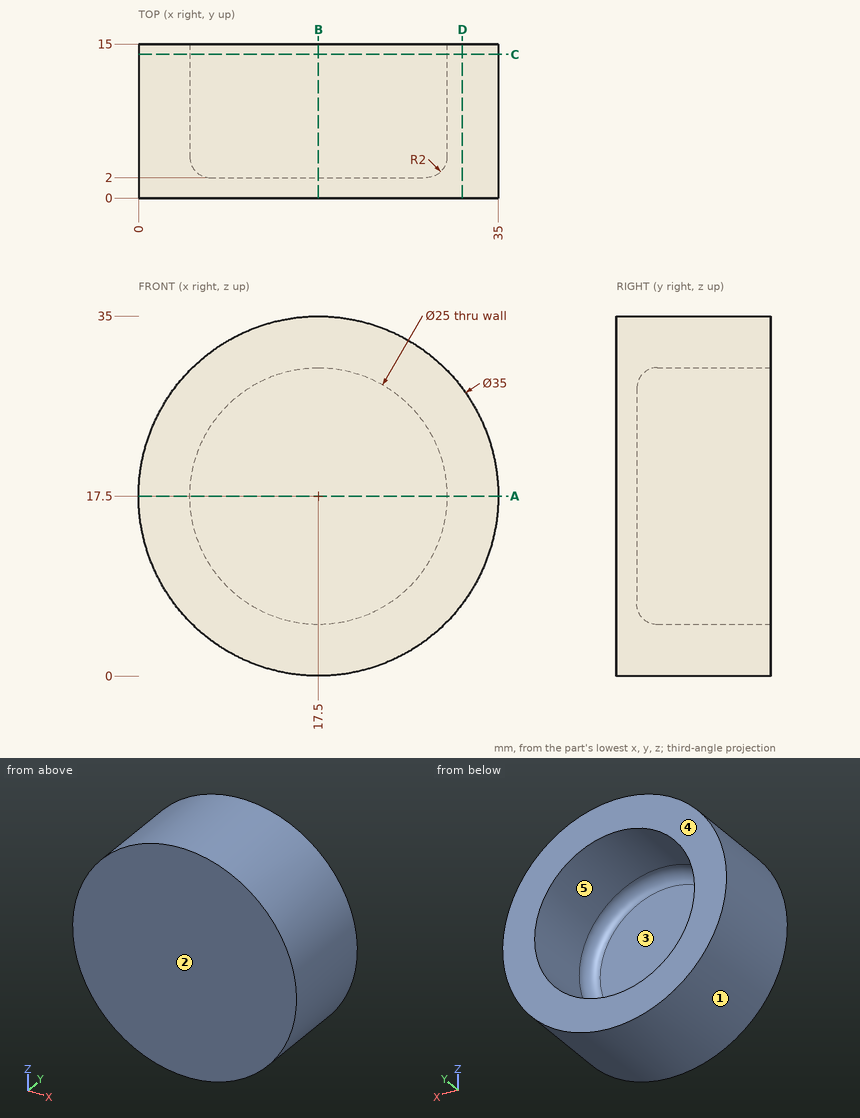
Can you work these out from the drawing? Everything is in mm from the part's minimum corner. A direction names the side the tool comes from. Give positions to 0.01 mm unless a question says otherwise; leave off trailing zeros. Order: outer loops, then holes, each group sorted by start corner. A loop starts at its lowest first (then second) coordinate and runs counter-clockwise, first axis right, second up.
1. For the marked faces 4 and 5, which set-ups out of +Z, -Z, +X, -X, +Y, -Y let a thin tool reach every point of the face, with its end or its side?
2. Suppose I cut it at C-C (y = 14). List the corners of the cut face in (x, z) for me.
3. We'd pull the mould along X, two halves only. Please class the marked faces 1, 2 and 3: pulls with the +X half, pulls with the -X half, needs draft (parallel to the pull), parting line crosses it, or undercut.
4. Suppose I cut it at D-D (x = 31.5). List the corners of the cut face in (y, z) for me, plus the area to 3 significant figures.
5. Suppose I cut it at A-A (z = 17.5). List the corners of the cut face in (x, y) for me.
6. I need wall thicknesses on L1, parallel to X at y = 9.75, z = 17.5; L2, parallel to Y at x = 12.5, z = 24; L3, parallel to Z at x = 24, y = 13. Which ranges of each line are inside material? Lowest first, please.
7. Will these pins go through, and if not, where does the flat tip stop? P1, Ø8, axis at y = 3, z = 4.5, coming from the -X side; P2, Ø1, axis at x = 22.5, y = 5.5, coming from the -Z side; P3, Ø6, axis at x = 13, y = 13, coming from the -Z side.
8. Suppose I cut it at B-B (x = 17.5). List the corners of the cut face in (y, z) for me, plus the area to 3 significant figures.
Solved:
1. face 4: +Z, -Z, +X, -X, +Y
1. face 5: +Y
2. outline: circle Ø35 at (17.5, 17.5); hole circle Ø25 at (17.5, 17.5)
3. face 1: parting line crosses it
3. face 2: needs draft
3. face 3: undercut
4. outline: (0, 7) - (15, 7) - (15, 28) - (0, 28) - close
4. area: 315 mm2
5. outline: (0, 0) - (35, 0) - (35, 15) - (30, 15) - (30, 4) arc R2 cw to (28, 2) - (7, 2) arc R2 cw to (5, 4) - (5, 15) - (0, 15) - close
6. L1: x = 0 to 5, 30 to 35
6. L2: y = 0 to 2
6. L3: z = 1.25 to 6.82, 28.18 to 33.75
7. P1: stops at x = 2.49
7. P2: stops at z = 0.59
7. P3: stops at z = 0.06
8. outline: (0, 0) - (15, 0) - (15, 5) - (4, 5) arc R2 cw to (2, 7) - (2, 28) arc R2 cw to (4, 30) - (15, 30) - (15, 35) - (0, 35) - close
8. area: 202 mm2
